Autodesk Inventor part; units mm, degrees
ref_plane "YZ Plane" through (0, 0, 0) normal (1, 0, 0) x (0, 1, 0)
ref_plane "XZ Plane" through (0, 0, 0) normal (0, 1, 0) x (-1, 0, 0)
ref_plane "XY Plane" through (0, 0, 0) normal (0, 0, 1) x (1, 0, 0)
sketch "Sketch1" plane through (0, 0, 0) normal (0, 0, 1) x (1, 0, 0)
  circle A0 centre (0, 0) radius 7.9375
  dimension "d0" = 15.875
extrude "Extrusion1" add sketch "Sketch1" along normal mid plane 90.4875
sketch "Sketch2" plane through (0, 0, 45.2437) normal (0, 0, 1) x (1, 0, 0)
  line L0 (-3.6662, 6.35) -> (3.6662, 6.35)
  line L1 (3.6662, 6.35) -> (7.3323, 0)
  line L2 (7.3323, 0) -> (3.6662, -6.35)
  line L3 (3.6662, -6.35) -> (-3.6662, -6.35)
  line L4 (-3.6662, -6.35) -> (-7.3323, 0)
  line L5 (-7.3323, 0) -> (-3.6662, 6.35)
  circle A0 centre (0, 0) radius 7.9375
  point P0 (0, -6.35)
  point P1 (0, 6.35)
  dimension "d3" = 12.7
extrude "Extrusion2" cut sketch "Sketch2" against normal blind 53.975
sketch "Sketch3" plane through (0, 0, 45.2437) normal (0, 0, 1) x (1, 0, 0)
  circle A0 centre (0, 0) radius 6.35
  circle A1 centre (0, 0) radius 7.9375
  line L0 (3.6662, 6.35) -> (-3.6662, 6.35)
  line L1 (7.3323, 0) -> (3.6662, 6.35)
  line L2 (3.6662, -6.35) -> (7.3323, 0)
  line L3 (-3.6662, -6.35) -> (3.6662, -6.35)
  line L4 (-7.3323, 0) -> (-3.6662, -6.35)
  line L5 (-3.6662, 6.35) -> (-7.3323, 0)
  point P0 (-5.4993, 3.175)
  point P1 (0, 6.35)
  point P2 (-5.4993, -3.175)
  point P3 (0, -6.35)
  point P4 (5.4993, -3.175)
  point P5 (5.4993, 3.175)
  dimension "d6" = 12.7
extrude "Extrusion3" cut sketch "Sketch3" against normal blind 6.35 contours A0 L1 L2 | A0 L0 L1 | L2 L3 A0 | A0 L5 L0 | L3 L4 A0 | A0 L4 L5
sketch "Sketch6" plane through (0, 0, 0) normal (1, 0, 0) x (0, 1, 0)
  line L0 (7.9375, -45.2437) -> (-7.9375, -45.2437) construction
  line L1 (-7.9375, -45.2437) -> (-7.9375, -8.7312) construction
  line L2 (-7.9375, -8.7312) -> (-6.35, -8.7312) construction
  line L3 (-6.35, -8.7312) -> (-6.35, 38.8938) construction
  line L4 (-6.35, 38.8938) -> (-6.35, 45.2437) construction
  line L5 (-6.35, 45.2437) -> (6.35, 45.2437) construction
  line L6 (6.35, 45.2437) -> (6.35, 38.8938) construction
  line L7 (6.35, 38.8938) -> (6.35, -8.7312) construction
  line L8 (6.35, -8.7312) -> (7.9375, -8.7312) construction
  line L9 (7.9375, -8.7312) -> (7.9375, -45.2437) construction
  line L10 (6.35, 45.2437) -> (-6.35, 45.2437)
  line L11 (-6.35, 45.2437) -> (-6.35, 35.7187)
  line L12 (-6.35, 35.7187) -> (6.35, 35.7188)
  line L13 (6.35, 35.7188) -> (6.35, 45.2437)
  line L14 (7.9375, -45.2437) -> (-7.9375, -45.2437)
  line L15 (-7.9375, -45.2437) -> (-7.9375, -44.6088)
  line L16 (-7.9375, -44.6088) -> (7.9375, -44.6088)
  line L17 (7.9375, -44.6088) -> (7.9375, -45.2437)
  point P0 (0, 0)
  dimension "d15" = 9.525
  dimension "d16" = 0.635
extrude "Extrusion6" cut sketch "Sketch6" along normal through all both and the other way through all
sketch "Sketch7" plane through (0, 0, -44.6088) normal (0, 0, -1) x (-1, 0, 0)
  circle A0 centre (0, 0) radius 6.35
  circle A1 centre (0, 0) radius 7.9375
  circle A2 centre (0, 0) radius 7.9375 construction
  dimension "d19" = 12.7
extrude "Extrusion7" cut sketch "Sketch7" against normal blind 7.9375
properties part number "EL2-C2-002" material "Aluminum 6061"
The model under review builds one solid part; all positions refer to its coordinate system, in mm. A direction names the side the tool comes from. Give positions to 0.01 mm unless a question says otherwise; leave off trailing zeros. Write each loop counter-clockwise with the first axis right and the second up, starting at its lowest first coordinate (ties: lowest second). Pieces come first, ordered by that corner, then holes. Notation, with made-up numbers: (-31, 0) -> (11, 0) arc R18 ccw to (11, 8) -> close; hole circle Ø11 at (-30, 43). An arc over 180 degrees is marked (long way). Answer in a Markdown table with one row per item.
1) For L1, parallel to Y at x = -1.75, z = 8.5; L2, parallel to Z at x = -0.5, y = 6.5; L3, parallel to Y at x = -0.25, z = -30.5, list the stretches that pass through material, from the lowest coordinate up. Write a range as [from, to].
Worked answers:
| item | result |
|---|---|
| L1 | [-6.35, 6.35] |
| L2 | [-36.67, -8.73] |
| L3 | [-7.93, 7.93] |
2) Clearance check with flat-ended pins moving along their axes: P1, Ø5, axis at y = 5.5, z = -33.5, coming from the +X side; P2, Ø5, axis at x = 1, z = 3.5, coming from the +Y side; P3, Ø1, axis at x = 2, z = -19.5, coming from the +Y side. State where each tip first meets the part, or that it passes through.
Worked answers:
| item | result |
|---|---|
| P1 | x = 7.35 |
| P2 | y = 6.35 |
| P3 | y = 7.79 |
3) Add section C-C on y = 5. State the section outline as (x, z) points.
Worked answers:
| item | result |
|---|---|
| outline | (-6.16, -36.67) -> (-3.91, -36.67) -> (-3.91, -44.61) -> (3.91, -44.61) -> (3.91, -36.67) -> (6.16, -36.67) -> (6.16, -8.73) -> (4.45, -8.73) -> (4.45, 35.72) -> (-4.45, 35.72) -> (-4.45, -8.73) -> (-6.16, -8.73) -> close |
4) Tool access review of faces 1 (the flat face through (-5.474, -3.219, 13.805)), 2 (the flat face through (0, 6.35, 14)), 3 (the flat face through (5.525, -3.131, 13.805)), 4 (the flat face through (5.474, 3.219, 13.805)), 5 (the flat face through (-5.525, 3.131, 13.805)): name each direction out of +Z, -Z, +X, -X, +Y, -Y from which nothing blocks a thin tool from reaching the whole face with its end or side.
Worked answers:
| item | result |
|---|---|
| face 1 | +Z, -X, -Y |
| face 2 | +Z, +X, -X, +Y |
| face 3 | +Z, +X, -Y |
| face 4 | +Z, +X, +Y |
| face 5 | +Z, -X, +Y |
5) Add section A-A on x = 0. State the section outline as (y, z) points, plus the area to 3 significant figures.
Worked answers:
| item | result |
|---|---|
| outline | (-7.94, -36.67) -> (-6.35, -36.67) -> (-6.35, -44.61) -> (6.35, -44.61) -> (6.35, -36.67) -> (7.94, -36.67) -> (7.94, -8.73) -> (6.35, -8.73) -> (6.35, 35.72) -> (-6.35, 35.72) -> (-6.35, -8.73) -> (-7.94, -8.73) -> close |
| area | 1,110 mm² |
6) Add section D-D on z = -12. State the section outline as (x, y) points (1 decimal), plus the area to 3 significant figures.
Worked answers:
| item | result |
|---|---|
| outline | circle Ø15.9 at (0, 0) |
| area | 198 mm² |
7) Add section B-B on z = 1.5. State the section outline as (x, y) points.
Worked answers:
| item | result |
|---|---|
| outline | (-7.33, 0) -> (-3.67, -6.35) -> (3.67, -6.35) -> (7.33, 0) -> (3.67, 6.35) -> (-3.67, 6.35) -> close |
